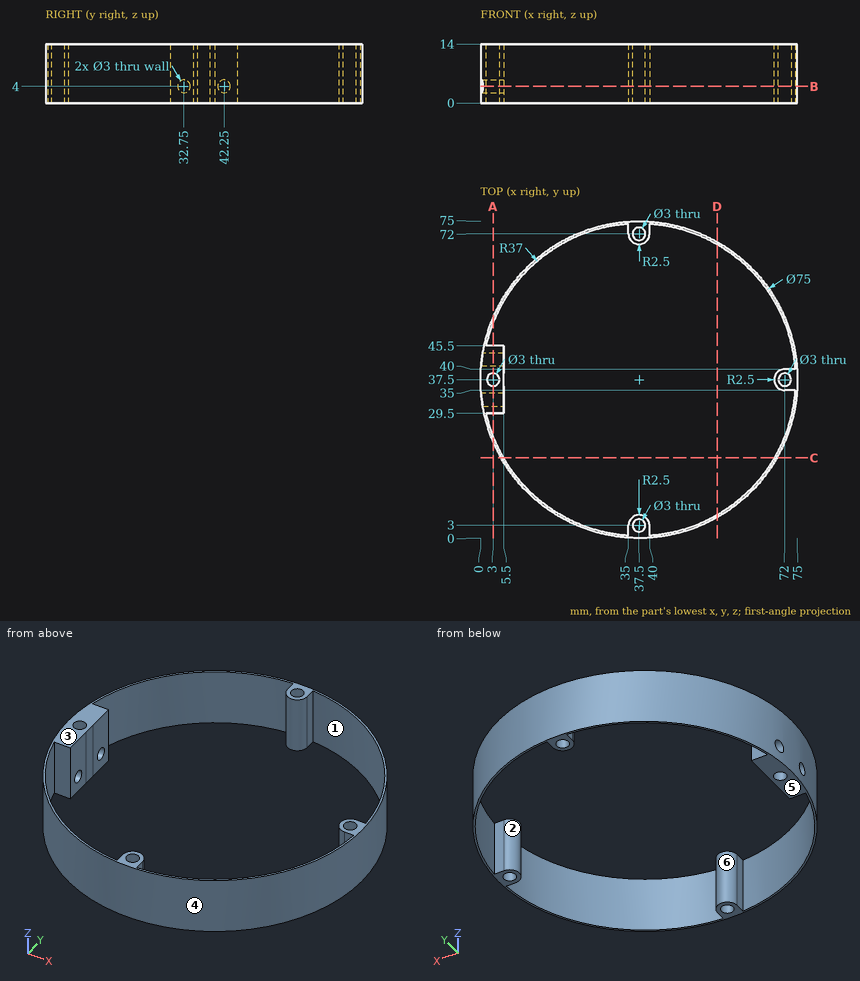
Design review of the part shown in the three views and the two pictorial views. Dimensions are in mm from the part's minimum x, y and z. A direction names the side the tool comes from. Coordinates: 2 decimals unless noted, no trailing zeros. Write each loop counter-clockwise with the first axis right and the second up, starting at its lowest first coordinate (ties: lowest second). Pieces come first, ordered by that corner, then holes.
1) Machinability: for the marked faces 5 and 6, which of the approach directions +Z, -Z, +X, -X, +Y, -Y give a long, thin tool a straight path to every point of the face, cutting with its end or side? Answer none if there is none.
2) We need section A-A on x = 3. State the section outline as (y, z) points.
3) The part is to be moulded in two halves that separate along Y. For the marked faces 1, 2, 3 and 4, say which applies: pulls with the +Y half, pulls with the -Y half, needs draft (parallel to the pull), parting line crosses it, or undercut.
4) We need section C-C on y = 19. State the section outline as (x, z) points.
5) Clearance check with flat-ended pins moving along their axes: pin 1 Ø3.5 at (y, z) = (42.25, 4) entering from -X; pin 2 Ø1 at (y, z) = (12.5, 9.5) entering from +X; pin 3 Ø3 at (x, y) = (9.5, 8.5) entering from -Z; pin 4 Ø3.5 at (x, z) = (3, 4.5) entering from -Y. State where each tip first meets the part, or that it passes through.
6) To check wall thickness, follow probe 1 along Y at (x, z) = (37.5, 6); probe 2 along Y at (x, z) = (37, 3); probe 3 along X at (y, z) = (37, 4). State the ranges of each line that lie inside material, in increasing order.
7) We need section B-B on z = 4. Count the separate pieces of the cut face and the enclosed holes in it, then the cut area to 3 significant figures.
Answer list:
1. face 5: -Z, +X, -X, +Y, -Y
1. face 6: +Z, -Z
2. outline: (22.8, 0) - (24.13, 0) - (24.13, 14) - (22.8, 14) - close; (29.5, 0) - (36, 0) - (36, 14) - (29.5, 14) - close; (39, 0) - (45.5, 0) - (45.5, 14) - (39, 14) - close; (50.87, 0) - (52.2, 0) - (52.2, 14) - (50.87, 14) - close; hole circle Ø3 at (32.75, 4); hole circle Ø3 at (42.25, 4)
3. face 1: undercut
3. face 2: undercut
3. face 3: needs draft
3. face 4: parting line crosses it
4. outline: (4.88, 0) - (5.46, 0) - (5.46, 14) - (4.88, 14) - close; (69.54, 0) - (70.12, 0) - (70.12, 14) - (69.54, 14) - close
5. pin 1: stops at x = 0.12
5. pin 2: stops at x = 65.89
5. pin 3: passes through
5. pin 4: stops at y = 19.23
6. probe 1: y = 0 to 1.5, 4.5 to 5.5, 69.5 to 70.5, 73.5 to 75
6. probe 2: y = 0 to 1.59, 4.41 to 5.45, 69.55 to 70.59, 73.41 to 75
6. probe 3: x = 0 to 1.59, 4.41 to 5.5, 69.55 to 70.59, 73.41 to 75
7. separate pieces: 2
7. enclosed holes: 4
7. area: 200 mm2
